Can you work these out from the model? Positions are in its coordinate system, mm. A direction names the side the tool comes from. Give positions to 0.01 mm unless a question says otherwise; leave off trailing zeros. Loops run counter-clockwise (first coordinate to the right, second up) from the corner with the lowest first, then second, coordinate; pieces in that order, holes last. Notation, with made-up numbers: (70.25, -20) - (114.25, -20) arc R15 cw to (114.25, -2) - close; hole circle Ø6 at (38.25, 68.5). An arc over 180 degrees is marked (long way). Answer as a JSON object with one key per item and string values. Group by question number.
Item 1: Suppose I cut it at A-A on y = -20. Write out the boundary of the cut face in (x, z).
Item 2: Suppose I cut it at B-B on z = 15.25. Write out the boundary of the cut face in (x, y).
Item 3: Suppose I cut it at C-C on x = -33. Write out the boundary of the cut face in (y, z), and give its area (3 significant figures).
Item 4: Suppose I cut it at D-D on y = 4. Write out the boundary of the cut face in (x, z), and give its area (3 significant figures).
Item 5: Will this pin go through, and if not, where does the flat tip stop? pin 1 (10 mm diameter, centred on x = -31.5, z = 20, fed in from +Y).
Item 6: Thinking about a two-plate mould opening in X: for faces 1 (the flat face through (60, 1, 12)), 2 (the flat face through (-40, -44, 12)), 3 (the flat face through (-50, -70, 12)), 4 (the flat face through (-60, 1, 12)), which applies, pulls with the +X half, pulls with the -X half, needs draft (parallel to the pull), parting line crosses it, or undercut?
Item 7: Please list where these lines run through material, in increasing order: L1, parallel to X at y = 54.5, z = 13.5; L2, parallel to Y at x = -22, z = 7.75; L3, parallel to Z at x = 30, y = -9.
Item 8: Which directions (+Z, -Z, +X, -X, +Y, -Y) give clear straight access to the entire face, cutting with the end or side of a thin tool? Please do faces 5 (the flat face through (50, 70, 12)), 6 (the flat face through (40, -44, 12)), 7 (the flat face through (0.8, 4.4, 16.7)), 8 (the flat face through (-1, 17.5, 12)), 9 (the flat face through (1, 1, 0)).
from build123d import *

# Parameters (mm, degrees)
F1_DEPTH = 25
F4_DEPTH = 166.4


with BuildPart() as f1:
    # F0 (on Top) → F1 (new body)
    with BuildSketch(Plane.XY):
        Polygon((-40, 17.5), (-40, 70), (-60, 70), (-60, -70), (-40, -70), (-40, -17.5), (0, -17.5), (0, 4.859984), (0, 17.5), align=None)
    extrude(amount=F1_DEPTH)

    # F2: F1 across plane


with BuildPart() as f1_1:
    add(f1.part)
    add(f1.part.mirror(Plane.YZ))

    # F3 (on face) → F4 (cut)
    with BuildSketch(Plane.YZ.offset(60)):
        Polygon((12.05619, 25), (0, 25), (-15.134365, 8.593241), (-3.078176, 8.593241), align=None)
    extrude(amount=-F4_DEPTH, mode=Mode.SUBTRACT)


solid = f1_1.part
Worked out:
{
 "1": {"outline": "(-60, 0) - (-40, 0) - (-40, 25) - (-60, 25) - close; (40, 0) - (60, 0) - (60, 25) - (40, 25) - close"},
 "2": {"outline": "(-60, -70) - (-40, -70) - (-40, -17.5) - (40, -17.5) - (40, -70) - (60, -70) - (60, -8.99) - (-60, -8.99) - close; (-60, 3.06) - (60, 3.06) - (60, 70) - (40, 70) - (40, 17.5) - (-40, 17.5) - (-40, 70) - (-60, 70) - close"},
 "3": {"outline": "(-17.5, 0) - (17.5, 0) - (17.5, 25) - (12.06, 25) - (-3.08, 8.59) - (-15.13, 8.59) - (0, 25) - (-17.5, 25) - close", "area": "677 mm2"},
 "4": {"outline": "(-60, 0) - (60, 0) - (60, 16.27) - (-60, 16.27) - close", "area": "1,950 mm2"},
 "5": {"pin 1": "stops at y = 17.5"},
 "6": {"face 1": "pulls with the +X half", "face 2": "undercut", "face 3": "needs draft", "face 4": "pulls with the -X half"},
 "7": {"L1": "x = -60 to -40, 40 to 60", "L2": "y = -17.5 to 17.5", "L3": "z = 0 to 8.59, 15.24 to 25"},
 "8": {"face 5": "+Z, -Z, +X, -X, +Y", "face 6": "+Z, -Z, -Y", "face 7": "+X, -X", "face 8": "+Z, -Z, +Y", "face 9": "-Z, +X, -X, +Y, -Y"}
}
